Work out the finished part from the listing and answer in its coordinate system (mm). Round coordinates to 2 decimals unless told otherwise and drop trailing zeros. Order: outer loops, then holes, each group sorted by start corner. A loop starts at its lowest first (then second) coordinate and runs counter-clockwise, first axis right, second up. Notation, with made-up numbers: (28, 46) -> (43, 46) arc R29 ccw to (43, 78) -> close; hole circle Ø4 at (45.5, -14.75). An arc over 180 degrees is marked (long way). Use a Markdown table: item, result. Add a question column.
Item 1: Find the intervals of material crossed by L1, parallel to Y at x = 6.65, z = 55; L2, parallel to X at y = -6.25, z = 101.5; L3, parallel to X at y = -13.45, z = 330, in increasing order. Write a range as [from, to].
Item 2: A cutting plane is placed at A-A, the plane y = -6. Determine the outline of the cut face in (x, z), plus the area to 3 significant figures.
Item 3: A cutting plane is placed at B-B, the plane z = 34. Determine the outline of the cut face in (x, y).
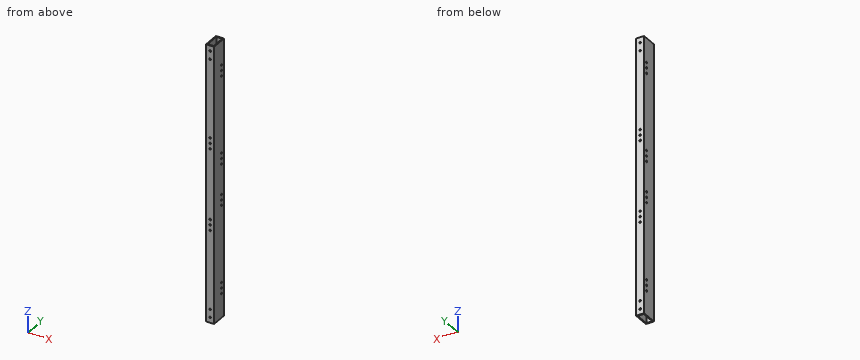
Autodesk Inventor part; units mm, degrees
ref_plane "YZ Plane" through (0, 0, 0) normal (1, 0, 0) x (0, 1, 0)
ref_plane "XZ Plane" through (0, 0, 0) normal (0, 1, 0) x (-1, 0, 0)
ref_plane "XY Plane" through (0, 0, 0) normal (0, 0, 1) x (1, 0, 0)
sketch "スケッチ1" plane through (0, 0, 0) normal (0, 0, 1) x (1, 0, 0)
  line L0 (7.5, 15) -> (-7.5, 15)
  line L1 (-7.5, 15) -> (-7.5, -15)
  line L2 (-7.5, -15) -> (7.5, -15)
  line L3 (7.5, -15) -> (7.5, 15)
  line L4 (7.5, 15) -> (-7.5, -15) construction
  line L5 (-7.5, 15) -> (7.5, -15) construction
  line L6 (-5.5, 13) -> (5.5, 13)
  line L7 (5.5, 13) -> (5.5, -13)
  line L8 (5.5, -13) -> (-5.5, -13)
  line L9 (-5.5, -13) -> (-5.5, 13)
  point P0 (0, 0)
  dimension "d0" = 15
  dimension "d1" = 30
  dimension "d2" = 2
extrude "押し出し1" add sketch "スケッチ1" along normal blind 510
sketch "スケッチ2" plane through (-7.5, 15, 0) normal (0, 1, 0) x (1, 0, 0)
  circle A0 centre (7.5, -10) radius 1.6
  circle A1 centre (7.5, -25) radius 1.6
  line L0 (15, 0) -> (0, 0)
  circle A2 centre (7.5, -500) radius 1.6
  circle A3 centre (7.5, -485) radius 1.6
  line L1 (15, -510) -> (0, -510)
  circle A4 centre (7.5, -170) radius 1.6
  circle A5 centre (7.5, -180) radius 1.6
  circle A6 centre (7.5, -190) radius 1.6
  circle A7 centre (7.5, -320) radius 1.6
  circle A8 centre (7.5, -330) radius 1.6
  circle A9 centre (7.5, -340) radius 1.6
  point P0 (7.5, 0)
  point P1 (7.5, 0)
  point P2 (7.5, -510)
  dimension "d5" = 3.2
  dimension "d6" = 3.2
  dimension "d7" = 10
  dimension "d8" = 15
  dimension "d9" = 3.2
  dimension "d10" = 3.2
  dimension "d11" = 10
  dimension "d12" = 15
  dimension "d15" = 3.2
  dimension "d16" = 3.2
  dimension "d17" = 3.2
  dimension "d18" = 10
  dimension "d19" = 10
  dimension "d20" = 180
  dimension "d21" = 3.2
  dimension "d22" = 3.2
  dimension "d23" = 3.2
  dimension "d24" = 10
  dimension "d25" = 10
  dimension "d26" = 180
extrude "押し出し2" cut sketch "スケッチ2" against normal through all
sketch "スケッチ3" plane through (7.5, -15, 0) normal (1, 0, 0) x (0, 0, -1)
  circle A0 centre (-293, 22.5) radius 1.6
  circle A1 centre (-283, 22.5) radius 1.6
  circle A2 centre (-303, 22.5) radius 1.6
  circle A3 centre (-217, 22.5) radius 1.6
  circle A4 centre (-207, 22.5) radius 1.6
  circle A5 centre (-227, 22.5) radius 1.6
  line L0 (-510, 0) -> (-510, 30)
  line L1 (0, 30) -> (-510, 30)
  circle A6 centre (-465, 22.5) radius 1.6
  circle A7 centre (-455, 22.5) radius 1.6
  circle A8 centre (-445, 22.5) radius 1.6
  circle A9 centre (-65, 22.5) radius 1.6
  circle A10 centre (-55, 22.5) radius 1.6
  circle A11 centre (-45, 22.5) radius 1.6
  point P0 (0, 15)
  dimension "d27" = 3.2
  dimension "d28" = 3.2
  dimension "d29" = 3.2
  dimension "d30" = 10
  dimension "d31" = 10
  dimension "d32" = 3.2
  dimension "d33" = 3.2
  dimension "d34" = 3.2
  dimension "d35" = 10
  dimension "d36" = 10
  dimension "d37" = 207
  dimension "d38" = 207
  dimension "d39" = 7.5
  dimension "d40" = 7.5
  dimension "d43" = 3.2
  dimension "d44" = 3.2
  dimension "d45" = 3.2
  dimension "d46" = 10
  dimension "d47" = 10
  dimension "d48" = 45
  dimension "d49" = 3.2
  dimension "d50" = 3.2
  dimension "d51" = 3.2
  dimension "d52" = 10
  dimension "d53" = 10
  dimension "d54" = 45
extrude "押し出し3" cut sketch "スケッチ3" against normal through all
properties part number "オムニ_角柱4" material "アルミニウム 6061"
Reported:
| question | item | result |
|---|---|---|
| 1 | L1 | [-15, 5.9], [9.1, 15] |
| 1 | L2 | [-7.5, -5.5], [5.5, 7.5] |
| 1 | L3 | [-7.5, -1.6], [1.6, 7.5] |
| 2 | outline | (-7.5, 0) -> (-5.5, 0) -> (-5.5, 510) -> (-7.5, 510) -> close; (5.5, 0) -> (7.5, 0) -> (7.5, 510) -> (5.5, 510) -> close |
| 2 | area | 2,040 mm² |
| 3 | outline | (-7.5, -15) -> (7.5, -15) -> (7.5, 15) -> (-7.5, 15) -> close; hole (-5.5, -13) -> (5.5, -13) -> (5.5, 13) -> (-5.5, 13) -> close |
